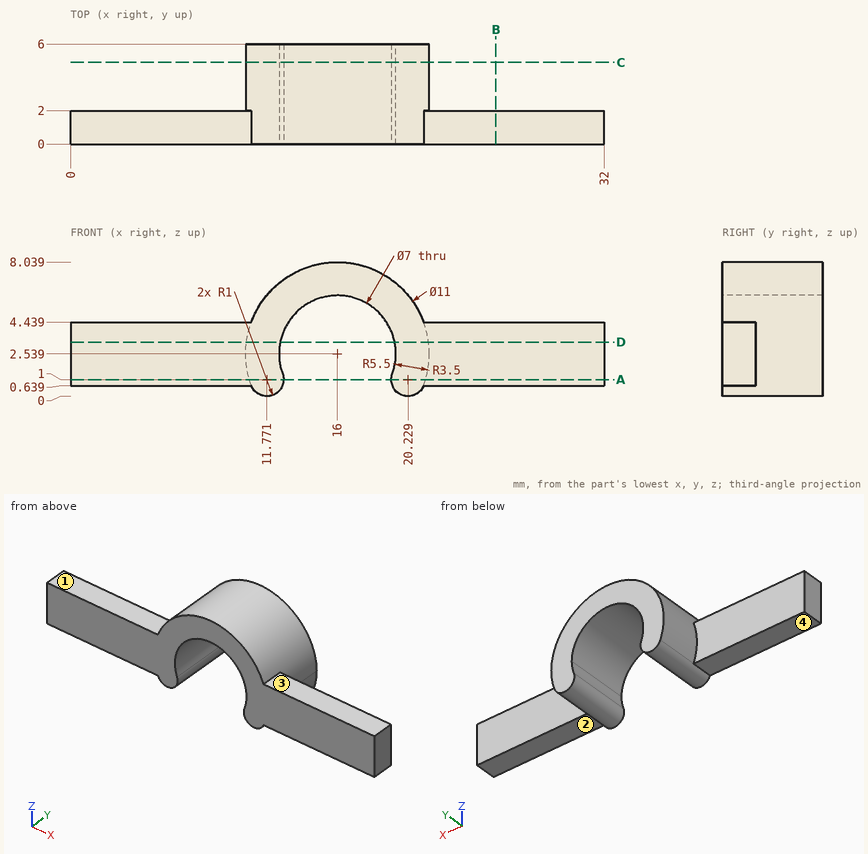
Part print with two shaded views. Sizes in mm from the minimum x, y, z corner. A direction names the side the tool comes from. Give positions to 0.01 mm unless a question says otherwise; leave off trailing zeros. Order: outer loops, then holes, each group sorted by start corner. A loop starts at its lowest first (then second) coordinate and runs counter-clockwise, first axis right, second up.
(1) Saw through at D-D, the plane z = 3.25. Give the cut face in (x, y).
(2) Saw through at B-B, the plane x = 25.5. Give the cut face in (y, z).
(3) Saw through at A-A, the plane z = 1. Give the cut face in (x, y).
(4) Saw through at C-C, the plane y = 4.9. Give the cut face in (x, z).
(5) Drill centre lines: L1, parallel to Z at x = 16, y = 2.4; L2, parallel to Y at x = 29.5, z = 3.25; L3, parallel to X at y = 4.25, z = 4.25. Where is each one in solid material? Low to high.
(6) Flat gauge pins, fed straight in: pin 1 (2 mm diameter, centred on x = 25.5, y = 1.5, fed in from +Z); pin 2 (2 mm diameter, centred on x = 27.5, y = 1, fed in from -Z); pin 3 (1 mm diameter, centred on y = 5, z = 5, fed in from +X). Where does each tip first touch, or does it go through?
(7) Tool access for the marked faces 1, 2, 3 and 4: list every direction of +Z, -Z, +X, -X, +Y, -Y with a clear straight run to the whole face (end or side of a thin tool).
Results found:
1. outline: (0, 0) - (12.57, 0) - (12.57, 6) - (10.55, 6) - (10.55, 2) - (0, 2) - close; (19.43, 0) - (32, 0) - (32, 2) - (21.45, 2) - (21.45, 6) - (19.43, 6) - close
2. outline: (0, 0.64) - (2, 0.64) - (2, 4.44) - (0, 4.44) - close
3. outline: (0, 0) - (12.77, 0) - (12.77, 6) - (10.72, 6) - (10.72, 2) - (0, 2) - close; (19.23, 0) - (32, 0) - (32, 2) - (21.28, 2) - (21.28, 6) - (19.23, 6) - close
4. outline: (10.83, 0.66) arc R1 ccw to (12.71, 1.34) arc R3.5 cw (long way) to (19.29, 1.34) arc R1 ccw to (21.17, 0.66) arc R5.5 ccw (long way) to start
5. L1: z = 6.04 to 8.04
5. L2: y = 0 to 2
5. L3: x = 10.77 to 12.95, 19.05 to 21.23
6. pin 1: stops at z = 4.44
6. pin 2: stops at z = 0.64
6. pin 3: stops at x = 21.14
7. face 1: +Z, -X, +Y, -Y
7. face 2: -Z, +X, +Y, -Y
7. face 3: +Z, +X, +Y, -Y
7. face 4: -Z, -X, +Y, -Y
